Autodesk Inventor part; units mm, degrees
ref_plane "YZ Plane" through (0, 0, 0) normal (1, 0, 0) x (0, 1, 0)
ref_plane "XZ Plane" through (0, 0, 0) normal (0, 1, 0) x (-1, 0, 0)
ref_plane "XY Plane" through (0, 0, 0) normal (0, 0, 1) x (1, 0, 0)
sketch "Sketch1" plane through (0, 0, 0) normal (0, 1, 0) x (-1, 0, 0)
  line L0 (0, 0) -> (19.4, 0)
  line L1 (19.4, 0) -> (19.4, -19.4)
  line L2 (19.4, -19.4) -> (0, -19.4)
  line L3 (0, -19.4) -> (0, 0)
  dimension "d0" = 19.4
  dimension "d1" = 19.4
extrude "Extrusion1" add sketch "Sketch1" along normal blind 3
sketch "Sketch2" plane through (0, 3, 0) normal (0, 1, 0) x (1, 0, 0)
  circle A0 centre (-15.8, 3.6) radius 1.6
  line L0 (-19.4, 19.4) -> (-19.4, 0)
  line L1 (-19.4, 0) -> (0, 0)
  dimension "d4" = 3.2
  dimension "d5" = 3.6
  dimension "d6" = 3.6
extrude "Extrusion2" cut sketch "Sketch2" against normal through all
pattern_linear "Rectangular Pattern1" count 2 spacing 12.2 along (0, 0, -1) count 2 spacing 12.2 along (1, 0, 0) of "Extrusion2"
sketch "Sketch3" plane through (0, 3, 0) normal (0, 1, 0) x (1, 0, 0)
  circle A0 centre (-9.7, 9.7) radius 5
  line L0 (-19.4, 0) -> (0, 0)
  line L1 (0, 0) -> (0, 19.4)
  dimension "d15" = 10
  dimension "d16" = 9.7
  dimension "d17" = 9.7
extrude "Extrusion3" add sketch "Sketch3" along normal blind 3
sketch "Sketch4" plane through (-9.7, 6, -9.7) normal (0, 1, 0) x (1, 0, 0)
  circle A0 centre (0, 0) radius 2.35
  line L0 (9.7, -9.7) -> (9.7, 9.7)
  line L1 (-9.7, -9.7) -> (9.7, -9.7)
  dimension "d20" = 4.7
  dimension "d21" = 9.7
  dimension "d22" = 9.7
extrude "Extrusion4" add sketch "Sketch4" along normal blind 10
fillet "Fillet1" radius 0.5 1 edges at (-14.7, 3, -9.7)
fillet "Fillet2" radius 0.5 1 edges at (-14.7, 6, -9.7)
fillet "Fillet3" radius 0.5 1 edges at (-12.05, 6, -9.7)
sketch "Sketch5" plane through (-9.7, 16, -9.7) normal (0, 1, 0) x (1, 0, 0)
  circle A0 centre (0, 0) radius 1.4
  line L0 (9.7, -9.7) -> (9.7, 9.7)
  line L1 (-9.7, -9.7) -> (9.7, -9.7)
  dimension "d28" = 2.8
  dimension "d29" = 9.7
  dimension "d30" = 9.7
extrude "Extrusion5" cut sketch "Sketch5" against normal through all
sketch "Sketch6" plane through (0, 3, 0) normal (0, 1, 0) x (1, 0, 0)
  circle A0 centre (-3.6, 3.6) radius 2.75
  line L0 (0, 0) -> (0, 19.4)
  line L1 (-19.4, 0) -> (0, 0)
  dimension "d33" = 5.5
  dimension "d34" = 3.6
  dimension "d35" = 3.6
extrude "Extrusion6" cut sketch "Sketch6" against normal blind 2
pattern_linear "Rectangular Pattern2" count 2 spacing 12.2 along (0, 0, -1) count 2 spacing 12.2 along (-1, 0, 0) of "Extrusion6"
sketch "Sketch7" plane through (0, 3, 0) normal (0, 1, 0) x (1, 0, 0)
  line L0 (-17.387, 18.55) -> (-14.2116, 18.55)
  line L1 (-14.2116, 18.55) -> (-12.6239, 15.8)
  line L2 (-12.6239, 15.8) -> (-14.2116, 13.05)
  line L3 (-14.2116, 13.05) -> (-17.387, 13.05)
  line L4 (-17.387, 13.05) -> (-18.9747, 15.8)
  line L5 (-18.9747, 15.8) -> (-17.387, 18.55)
  line L6 (-19.4, 19.4) -> (-19.4, 0)
  line L7 (0, 19.4) -> (-19.4, 19.4)
  point P0 (0, 0)
  dimension "d56" = 0
  dimension "d57" = 0
  dimension "d58" = 0
  dimension "d59" = 5.5
  dimension "d60" = 5.5
  dimension "d61" = 120
  dimension "d62" = 2.013
  dimension "d63" = 0.85
extrude "Extrusion7" cut sketch "Sketch7" against normal blind 2
pattern_linear "Rectangular Pattern3" count 2 spacing 12.3 along (1, 0, 0) count 2 spacing 12.2 along (0, 0, 1) of "Extrusion7"
chamfer "Chamfer1" distance 0.5 angle 45 1 edges at (-12.05, 16, -9.7)
equation "\"d1\" = d0"
equation "\"d17\" = d16"
properties part number "INTERFACE_MANIFOLD"
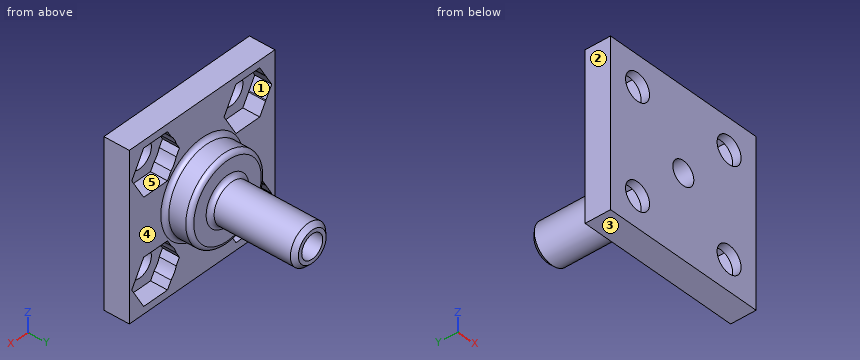
Geometry: final body of the model. Coordinates: model frame, mm. Face numbers are marked on the shaded views. A direction names the side the tool comes from. Round coordinates to 2 decimals unless told otherwise and drop trailing zeros. Loops run counter-clockwise (first coordinate to the right, second up) from the corner with the lowest first, then second, coordinate; pieces in that order, holes last. Notation, with made-up numbers: M 27.25,66 L 32.25,66 A16 cw 32.25,80 Z; hole C -22.75,5.5 d9. An arc over 180 degrees is marked long. One line per question, with ' | ' between items.
(1) Cut plane D-D on y = 8. Return the cut outline in (x, z), plus the area to 3 significant figures.
Check result:
outline: C -9.7,-9.7 d4.7; hole C -9.7,-9.7 d2.8 | area: 11.2 mm2
(2) Cut plane B-B on z = -9.7. Return the cut outline in (x, y), plus the area to 3 significant figures.
Check result:
outline: M -19.4,0 L -11.1,0 L -11.1,16 L -11.55,16 L -12.05,15.5 L -12.05,6.5 A0.5 cw -12.55,6 L -14.2,6 A0.5 ccw -14.7,5.5 L -14.7,3.5 A0.5 cw -15.2,3 L -19.4,3 Z; M -8.3,0 L 0,0 L 0,3 L -4.2,3 A0.5 cw -4.7,3.5 L -4.7,5.5 A0.5 ccw -5.2,6 L -6.85,6 A0.5 cw -7.35,6.5 L -7.35,15.5 L -7.85,16 L -8.3,16 Z | area: 90.3 mm2
(3) Cut plane A-A on x = -3.6. Return the cut outline in (y, z).
Check result:
outline: M 0,-19.4 L 3,-19.4 L 3,-18.55 L 1,-18.55 L 1,-17.4 L 0,-17.4 Z; M 0,-14.2 L 1,-14.2 L 1,-13.05 L 3,-13.05 L 3,-6.35 L 1,-6.35 L 1,-5.2 L 0,-5.2 Z; M 0,-2 L 1,-2 L 1,-0.85 L 3,-0.85 L 3,0 L 0,0 Z
(4) Access query for the marked faces 1 and 2. Directions: +Z, -Z, +X, -X, +Y, -Y. A direction counts if a zero-diameter tool reaches every point of the face in a straight line with its end or side. Return the directions, or none.
Check result:
face 1: +Y | face 2: +Z, -Z, -X, +Y, -Y
(5) Material intervals for line 1 along Z through (x, y) = (-15.8, 0.35); line 2 along Z through (x, y) = (-9.7, 12.5), sorted ascending. Write a range as from..to.
Check result:
line 1: z = -19.4..-17.4, -14.2..-5.2, -2..0 | line 2: z = -12.05..-11.1, -8.3..-7.35
(6) Cut plane C-C on x = -9.7. Return the cut outline in (y, z).
Check result:
outline: M 0,-19.4 L 3,-19.4 L 3,-15.2 A0.5 cw 3.5,-14.7 L 5.5,-14.7 A0.5 ccw 6,-14.2 L 6,-12.55 A0.5 cw 6.5,-12.05 L 15.5,-12.05 L 16,-11.55 L 16,-11.1 L 0,-11.1 Z; M 0,-8.3 L 16,-8.3 L 16,-7.85 L 15.5,-7.35 L 6.5,-7.35 A0.5 cw 6,-6.85 L 6,-5.2 A0.5 ccw 5.5,-4.7 L 3.5,-4.7 A0.5 cw 3,-4.2 L 3,0 L 0,0 Z
(7) Contact query for flat-ended pins moving along their axis: P1, Ø8, axis at x = -11, y = 10.5, coming from the +Z side; P2, Ø1, axis at x = -3, y = 7, coming from the +Z side; P3, Ø3, axis at x = -16.5, z = -2.5, coming from the +Y side; P4, Ø4.5, axis at x = -4.5, z = -16.5, coming from the +Y side. Output: stop coordinate, or through.
Check result:
P1: stops at z = -7.35 | P2: passes through | P3: stops at y = 1 | P4: stops at y = 3
(8) Pull-direction query (Z, two-part tool) for the marked faces 3, 4 and 5; classes: +Z half, -Z half, draft (parallel to the pull), parting line (faces both ways), or undercut.
Check result:
face 3: -Z half | face 4: draft | face 5: undercut
